Here's how the part is built. I have some questions about the finished solid (model axes, mm). Face numbers are marked on the shaded views. A direction names the side the tool comes from. Round coordinates to 2 decimals unless told otherwise and drop trailing zeros. Write each loop counter-clockwise with the first axis right and the second up, starting at its lowest first coordinate (ties: lowest second). Pieces come first, ordered by that corner, then holes. Notation, with made-up numbers: M 4,42 L 9,42 A19 cw 9,48 Z; hole C -38,-17.5 d11. An arc over 180 degrees is marked long. Use a Markdown table: item, result. Add a question column.
```python
from build123d import *

# Parameters (mm, degrees)
SKETCH1_R           = 20
BOSS_EXTRUDE1_DEPTH = 3
SKETCH2_R           = 19.25
BOSS_EXTRUDE2_DEPTH = 2
SKETCH3_W           = 30
SKETCH3_H           = 30
BOSS_EXTRUDE3_DEPTH = 26.1


with BuildPart() as part:
    # Sketch1 → Boss-Extrude1 (new body)
    # profile 1 of 6: a face of its own
    with BuildSketch(Plane.XY):
        with BuildLine():
            Line((10.050373127, 23), (-10.050373127, 23))
            ThreePointArc((-10.050373127, 23), (-13.456072932, 21.188301047), (-16.54393585, 18.876127426))
            ThreePointArc((-16.54393585, 18.876127426), (-16.213806457, 18.354666777), (-16.098380208, 17.748380208))
            ThreePointArc((-16.098380208, 17.748380208), (-17.091982047, 16.234563358), (-18.876127426, 16.54393585))
            ThreePointArc((-18.876127426, 16.54393585), (-21.188301047, 13.456072932), (-23, 10.050373127))
            Line((-23, 10.050373127), (-23, -10.050373127))
            ThreePointArc((-23, -10.050373127), (-21.188301047, -13.456072932), (-18.876127426, -16.54393585))
            ThreePointArc((-18.876127426, -16.54393585), (-17.091982047, -16.234563358), (-16.098380208, -17.748380208))
            ThreePointArc((-16.098380208, -17.748380208), (-16.213806457, -18.354666777), (-16.54393585, -18.876127426))
            ThreePointArc((-16.54393585, -18.876127426), (-13.456072932, -21.188301047), (-10.050373127, -23))
            Line((-10.050373127, -23), (10.050373127, -23))
            ThreePointArc((10.050373127, -23), (13.456072932, -21.188301047), (16.54393585, -18.876127426))
            ThreePointArc((16.54393585, -18.876127426), (16.581654019, -16.581654019), (18.876127426, -16.54393585))
            ThreePointArc((18.876127426, -16.54393585), (21.188301047, -13.456072932), (23, -10.050373127))
            Line((23, -10.050373127), (23, 10.050373127))
            ThreePointArc((23, 10.050373127), (21.188301047, 13.456072932), (18.876127426, 16.54393585))
            ThreePointArc((18.876127426, 16.54393585), (16.581654019, 16.581654019), (16.54393585, 18.876127426))
            ThreePointArc((16.54393585, 18.876127426), (13.456072932, 21.188301047), (10.050373127, 23))
        make_face()
        Circle(SKETCH1_R, mode=Mode.SUBTRACT)
    # profile 2 of 6: a face of its own
    with BuildSketch(Plane.XY):
        Circle(SKETCH1_R)
    # profile 3 of 6: a face of its own
    with BuildSketch(Plane.XY):
        with BuildLine():
            Line((23, 23), (10.050373127, 23))
            ThreePointArc((10.050373127, 23), (13.456072932, 21.188301047), (16.54393585, 18.876127426))
            ThreePointArc((16.54393585, 18.876127426), (18.354666777, 19.282953958), (19.398380208, 17.748380208))
            ThreePointArc((19.398380208, 17.748380208), (19.262197058, 17.091982047), (18.876127426, 16.54393585))
            ThreePointArc((18.876127426, 16.54393585), (21.188301047, 13.456072932), (23, 10.050373127))
            Line((23, 10.050373127), (23, 23))
        make_face()
    # profile 4 of 6: a face of its own
    with BuildSketch(Plane.XY):
        with BuildLine():
            Line((-10.050373127, 23), (-23, 23))
            Line((-23, 23), (-23, 10.050373127))
            ThreePointArc((-23, 10.050373127), (-21.188301047, 13.456072932), (-18.876127426, 16.54393585))
            ThreePointArc((-18.876127426, 16.54393585), (-18.915106397, 18.915106397), (-16.54393585, 18.876127426))
            ThreePointArc((-16.54393585, 18.876127426), (-13.456072932, 21.188301047), (-10.050373127, 23))
        make_face()
    # profile 5 of 6: a face of its own
    with BuildSketch(Plane.XY):
        with BuildLine():
            Line((23, -23), (23, -10.050373127))
            ThreePointArc((23, -10.050373127), (21.188301047, -13.456072932), (18.876127426, -16.54393585))
            ThreePointArc((18.876127426, -16.54393585), (19.262197058, -17.091982047), (19.398380208, -17.748380208))
            ThreePointArc((19.398380208, -17.748380208), (18.354666777, -19.282953958), (16.54393585, -18.876127426))
            ThreePointArc((16.54393585, -18.876127426), (13.456072932, -21.188301047), (10.050373127, -23))
            Line((10.050373127, -23), (23, -23))
        make_face()
    # profile 6 of 6: a face of its own
    with BuildSketch(Plane.XY):
        with BuildLine():
            ThreePointArc((-18.876127426, -16.54393585), (-21.188301047, -13.456072932), (-23, -10.050373127))
            Line((-23, -10.050373127), (-23, -23))
            Line((-23, -23), (-10.050373127, -23))
            ThreePointArc((-10.050373127, -23), (-13.456072932, -21.188301047), (-16.54393585, -18.876127426))
            ThreePointArc((-16.54393585, -18.876127426), (-18.915106397, -18.915106397), (-18.876127426, -16.54393585))
        make_face()
    extrude(amount=BOSS_EXTRUDE1_DEPTH)

    # Sketch2 → Boss-Extrude2 (add)
    with BuildSketch(Plane.XY.offset(3)):
        Circle(SKETCH2_R)
    extrude(amount=BOSS_EXTRUDE2_DEPTH)

    # Sketch3 → Boss-Extrude3 (add)
    with BuildSketch(Plane(origin=(0, 0, 0), x_dir=(-1, 0, 0), z_dir=(0, 0, -1))):
        Rectangle(SKETCH3_W, SKETCH3_H)
    extrude(amount=BOSS_EXTRUDE3_DEPTH)


solid = part.part
```
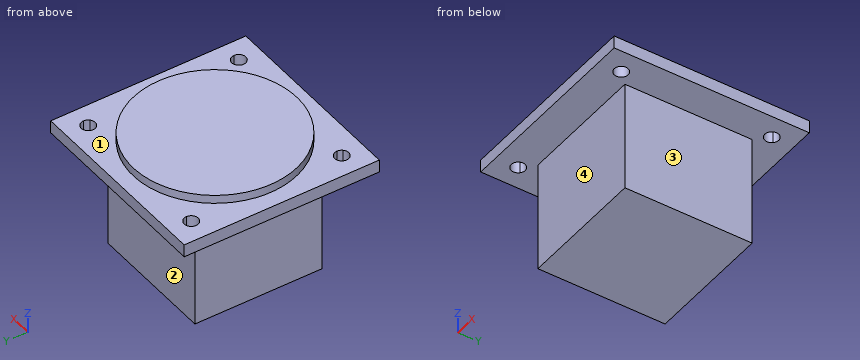
Item 1: I need wall thicknesses on probe 1 along Y at (x, z) = (-9, -9); probe 2 along Z at (x, y) = (-20, -14.5). Which ranges of each line are inside material? Lowest first, please. Write a range as from..to.
Item 2: Imagine slicing it at C-C on z = -4.5. List the corners of the cut face in (x, y) for me.
Item 3: For pin 1 Ø13 at (x, z) = (-6.5, -10) entering from +Y; pin 2 Ø5 at (y, z) = (-2, -9.5) entering from -X; pin 3 Ø1 at (x, y) = (-14, 16) entering from -Z; pin 4 Ø6 at (x, y) = (-16.5, -10) entering from -Z, each with a flat end and sliding along its axis, tell me the tip position at first contact or that it passes through.
Item 4: Imagine slicing it at D-D on y = 20. List the corners of the cut face in (x, z) for me, plus the area to 3 significant figures.
Item 5: Imagine slicing it at A-A on x = 0. List the corners of the cut face in (y, z) for me.
Item 6: On a 3-axis mill with a long thin cutter (end or side, diameter ignored), from which of +Z, -Z, +X, -X, +Y, -Y can I reach the whole of each face in a straight line? I mean the marked faces 1, 2, 3 and 4. Say none if no direction works.
The answers:
| question | item | result |
|---|---|---|
| 1 | probe 1 | -15..15 |
| 1 | probe 2 | 0..3 |
| 2 | outline | M -15,-15 L 15,-15 L 15,15 L -15,15 Z |
| 3 | pin 1 | y = 15 |
| 3 | pin 2 | x = -15 |
| 3 | pin 3 | z = 0 |
| 3 | pin 4 | z = -26.1 |
| 4 | outline | M -23,0 L 23,0 L 23,3 L -23,3 Z |
| 4 | area | 138 mm² |
| 5 | outline | M -23,0 L -15,0 L -15,-26.1 L 15,-26.1 L 15,0 L 23,0 L 23,3 L 19.25,3 L 19.25,5 L -19.25,5 L -19.25,3 L -23,3 Z |
| 6 | face 1 | +Z |
| 6 | face 2 | -Z, +X, -X, +Y |
| 6 | face 3 | -Z, +X, +Y, -Y |
| 6 | face 4 | -Z, +X, -X, -Y |
